The model under review builds one solid part; all positions refer to its coordinate system, in mm. Coordinates: 2 decimals unless noted, no trailing zeros. Loops run counter-clockwise (first coordinate to the right, second up) from the corner with the lowest first, then second, coordinate; pieces in that order, holes last. Notation, with made-up numbers: M 86,67 L 109,67 A32 cw 109,93 Z; hole C 72.5,-30 d7. An arc over 180 degrees is marked long. Use CSV: the item, a comma, the result in double quotes. Start each with the question number.
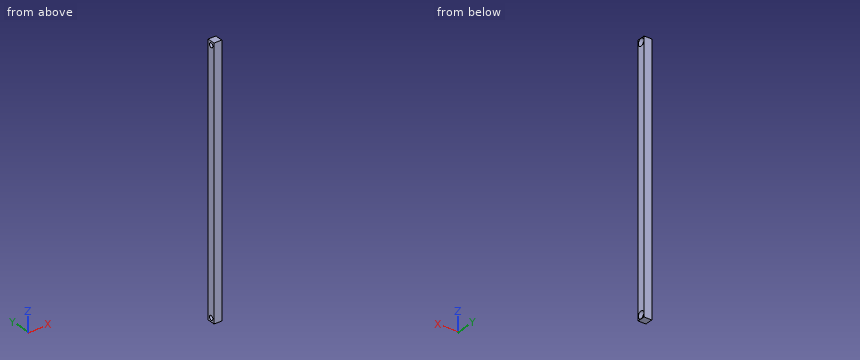
from build123d import *

# Parameters (mm, degrees)
IZIM1_W                     = 15
IZIM1_H                     = 15
Y_KSEKLIK_EKSTR_ZYON1_DEPTH = 252.5
DELIK2_D                    = 8.5
DELIK2_DEPTH                = 15
DELIK2_CBORE_D              = 14
DELIK2_CBORE_DEPTH          = 8


with BuildPart() as part:
    # Çizim1 → Yükseklik-Ekstrüzyon1 (new body, symmetric)
    with BuildSketch(Plane.XY):
        Rectangle(IZIM1_W, IZIM1_H)
    extrude(amount=Y_KSEKLIK_EKSTR_ZYON1_DEPTH, both=True)

    # Delik2
    with Locations(Plane(origin=(7.5, 0, 0), x_dir=(0, 0, -1), z_dir=(1, 0, 0))):
        with Locations((245, 0)):
            delik2 = CounterBoreHole(DELIK2_D / 2, DELIK2_CBORE_D / 2, DELIK2_CBORE_DEPTH, depth=DELIK2_DEPTH)

    # Aynalama1: Delik2 across plane
    add(delik2.mirror(Plane.XY), mode=Mode.SUBTRACT)


solid = part.part
1. Insertion check: pin 1 Ø4 at (y, z) = (2.5, -245.5) entering from +X. The pin has a flat end and moves straight along its axis. Give the tip position at first contact, or say it passes through.
2. Add section A-A (z = 245). Write out the cut boundary in (x, y).
3. Add section C-C (x = 3.25). Write out the cut boundary in (y, z).
4. To check wall thickness, follow line 1 along Z through (x, y) = (-6.5, -0.5); line 2 along Y through (x, z) = (2.25, -245); line 3 along Z through (x, y) = (2, 4.25). State the ranges of each line that lie inside material, in increasing order.
5. Add section B-B (y = 0). Write out the cut boundary in (x, z), plus the area to 3 significant figures.
Solved:
1,pin 1,"stops at x = -0.5"
2,outline,"M -7.5,-7.5 L 7.5,-7.5 L 7.5,-7 L -0.5,-7 L -0.5,-4.25 L -7.5,-4.25 Z; M -7.5,4.25 L -0.5,4.25 L -0.5,7 L 7.5,7 L 7.5,7.5 L -7.5,7.5 Z"
3,outline,"M -7.5,-252.5 L 7.5,-252.5 L 7.5,252.5 L -7.5,252.5 Z; hole C 0,-245 d14; hole C 0,245 d14"
4,line 1,"z = -252.5 to -249.22, -240.78 to 240.78, 249.22 to 252.5"
4,line 2,"y = -7.5 to -7, 7 to 7.5"
4,line 3,"z = -252.5 to -250.56, -239.44 to 239.44, 250.56 to 252.5"
5,outline,"M -7.5,-252.5 L 7.5,-252.5 L 7.5,-252 L -0.5,-252 L -0.5,-249.25 L -7.5,-249.25 Z; M -7.5,-240.75 L -0.5,-240.75 L -0.5,-238 L 7.5,-238 L 7.5,238 L -0.5,238 L -0.5,240.75 L -7.5,240.75 Z; M -7.5,249.25 L -0.5,249.25 L -0.5,252 L 7.5,252 L 7.5,252.5 L -7.5,252.5 Z"
5,area,"7,230 mm^2"
